from build123d import *

# Parameters (mm, degrees)
SKETCH1_R           = 12.7
BOSS_EXTRUDE3_DEPTH = 152.4
SKETCH12_W          = 63.5
SKETCH12_H          = 63.5
BOSS_EXTRUDE5_DEPTH = 10.16
SKETCH9_R           = 6.35
BOSS_EXTRUDE6_DEPTH = 19.05
SKETCH16_W          = 25.4
SKETCH16_H          = 63.5
CUT_EXTRUDE2_DEPTH  = 170.957130183
SKETCH17_W          = 25.4
SKETCH17_H          = 63.5
CUT_EXTRUDE3_DEPTH  = 170.957130183
SKETCH19_R          = 2.54
CUT_EXTRUDE5_DEPTH  = 170.957130183


with BuildPart() as part:
    # Sketch1 → Boss-Extrude3 (new, symmetric)
    with BuildSketch(Plane.XY):
        with Locations(Location((0, 0, 0), (0, 0, 180))):
            Circle(SKETCH1_R)
    extrude(amount=BOSS_EXTRUDE3_DEPTH, both=True)

    # Sketch12 → Boss-Extrude5 (add)
    with BuildSketch(Plane.XY.offset(152.4)):
        Rectangle(SKETCH12_W, SKETCH12_H)
    extrude(amount=BOSS_EXTRUDE5_DEPTH)

    # Sketch9 → Boss-Extrude6 (add, symmetric)
    with BuildSketch(Plane(origin=(0, 0, 0), x_dir=(0, 0, -1), z_dir=(1, 0, 0))):
        with Locations((-25.4, 0)):
            Circle(SKETCH9_R)
    extrude(amount=BOSS_EXTRUDE6_DEPTH, both=True)

    # Sketch16 → Cut-Extrude2 (cut, through all)
    with BuildSketch(Plane(origin=(0, -6.35, 0), x_dir=(1, 0, 0), z_dir=(0, 1, 0))):
        with Locations((0, 120.65)):
            Rectangle(SKETCH16_W, SKETCH16_H)
    extrude(amount=-CUT_EXTRUDE2_DEPTH, mode=Mode.SUBTRACT)

    # Sketch17 → Cut-Extrude3 (cut, through all)
    with BuildSketch(Plane(origin=(0, 6.35, 0), x_dir=(1, 0, 0), z_dir=(0, 1, 0))):
        with Locations((0, 120.65)):
            Rectangle(SKETCH17_W, SKETCH17_H)
    extrude(amount=CUT_EXTRUDE3_DEPTH, mode=Mode.SUBTRACT)

    # Sketch19 → Cut-Extrude5 (cut, through all)
    with BuildSketch(Plane(origin=(0, 6.35, 0), x_dir=(1, 0, 0), z_dir=(0, 1, 0))):
        with Locations(Location((0, 100.80625, 0), (0, 0, 270))):
            Circle(SKETCH19_R)
        with Locations(Location((0, 136.525, 0), (0, 0, 270))):
            Circle(SKETCH19_R)
    extrude(amount=-CUT_EXTRUDE5_DEPTH, mode=Mode.SUBTRACT)


solid = part.part
Could you check a few things on this model? Use its own coordinates, in mm. A direction names the side the tool comes from. Round coordinates to 2 decimals unless told otherwise and drop trailing zeros. Order: outer loops, then holes, each group sorted by start corner. A loop starts at its lowest first (then second) coordinate and runs counter-clockwise, first axis right, second up.
(1) Imagine slicing it at B-B (z = 25.4). Write out the boundary of the cut face in (x, y), plus the area to 3 significant figures.
Response values:
outline: (-19.05, -6.35) - (-11, -6.35) arc R12.7 ccw to (11, -6.35) - (19.05, -6.35) - (19.05, 6.35) - (11, 6.35) arc R12.7 ccw to (-11, 6.35) - (-19.05, 6.35) - close
area: 682 mm2
(2) Imagine slicing it at C-C (x = 25). Write out the boundary of the cut face in (y, z), plus the area to 3 significant figures.
Response values:
outline: (-31.75, 152.4) - (31.75, 152.4) - (31.75, 162.56) - (-31.75, 162.56) - close
area: 645 mm2
(3) Which directions (+Z, -Z, +X, -X, +Y, -Y) give clear straight access to the entire face, cutting with the end or side of a thin tool? Please do faces 1 (the flat face through (0, -9, -88.9)), 2 (the flat face through (19.05, 0, 25)), 3 (the cylindrical face through (15.08, -3.86, 30.44)).
Response values:
face 1: -Z, +X, -X, -Y
face 2: -Z, +X, +Y, -Y
face 3: +X
(4) Please list where these lines run through material, in increasing order: line 1 along Z through (x, y) = (-14, -0.5); line 2 along Z through (x, y) = (-23.5, 25.5); line 3 along X through (y, z) = (7.5, 2).
Response values:
line 1: z = 19.07 to 31.73, 152.4 to 162.56
line 2: z = 152.4 to 162.56
line 3: x = -10.25 to 10.25
(5) I'm going to push flat-ended pins straight in: pin 1 (1.9 mm diameter, centred on x = -2.5, y = -8.5, fed in from -Z); pin 2 (4 mm diameter, centred on y = -0.5, z = 24.5, fed in from +X); pin 3 (6.5 mm diameter, centred on x = -5, z = -110.5, fed in from -Y). Where does each tip first touch, or does it pass through?
Response values:
pin 1: stops at z = -88.9
pin 2: stops at x = 19.05
pin 3: stops at y = -6.35
(6) Imagine slicing it at A-A (y = 0). Write out the boundary of the cut face in (x, z) (3 decimals), plus the area to 3 significant figures.
Response values:
outline: (-31.75, 152.4) - (-12.7, 152.4) - (-12.7, 31.75) - (-19.05, 31.75) - (-19.05, 19.05) - (-12.7, 19.05) - (-12.7, -152.4) - (12.7, -152.4) - (12.7, 19.05) - (19.05, 19.05) - (19.05, 31.75) - (12.7, 31.75) - (12.7, 152.4) - (31.75, 152.4) - (31.75, 162.56) - (-31.75, 162.56) - close; hole circle Ø5.08 at (0, -136.525); hole circle Ø5.08 at (0, -100.806)
area: 8,510 mm2
(7) If we mould it in two halves opening along Z, with no side actions, what happens to faces 4 (the flat face through (-31.75, 0, 157)), 5 (the flat face through (0, 0, -152.4)), 6 (the cylindrical face through (-12.114, -3.815, 36))? For each: released by +Z, released by -Z, zero draft, split by the parting line, or undercut.
Response values:
face 4: zero draft
face 5: released by -Z
face 6: undercut
